Here's the drawing with two shaded views (mm, measured from the low corner). I have some questions. Coordinates: 2 decimals unless noted, no trailing zeros. Write each loop counter-clockwise with the first axis right and the second up, starting at its lowest first coordinate (ties: lowest second). Pieces come first, ordered by that corner, then holes.
Item 1: If we section it at A-A (x = 87.75): Please give me the cut outline in (y, z), then the cut area to 3 significant figures.
Item 2: If I drill on line 1 (Y direction, x = 87.75, z = 1.05); line 2 (Y direction, x = 2.2, z = 0.7); line 3 (Y direction, x = 4.75, z = 0.4), over which ranges is the centre line in solid material (lowest first)?
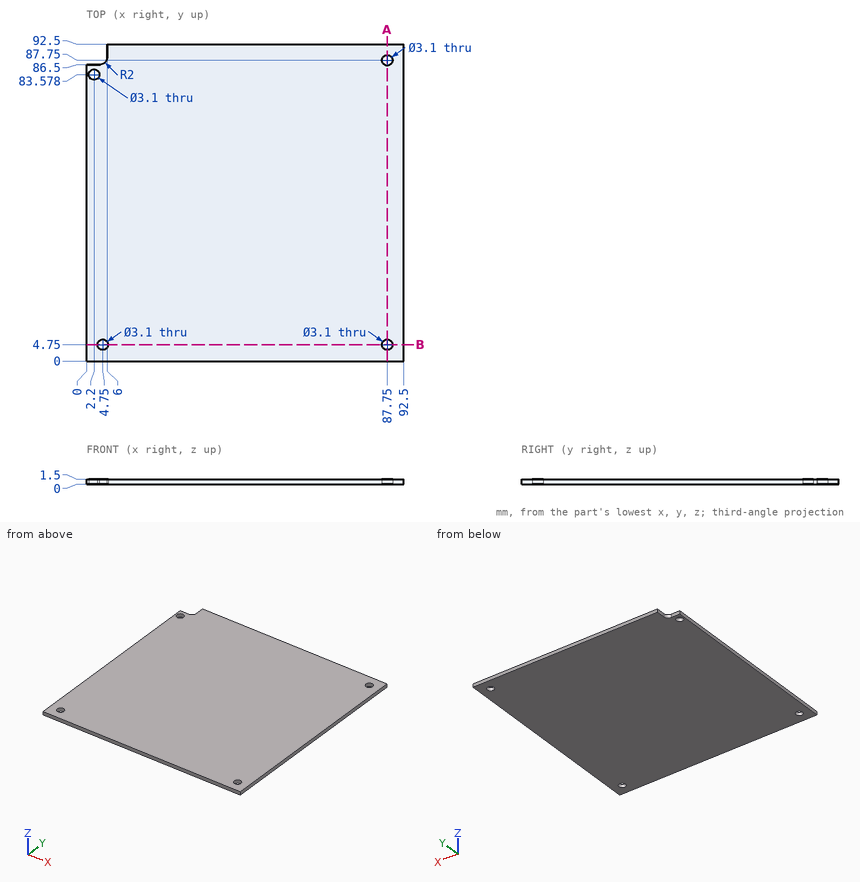
Answer list:
1. outline: (0, 0) - (3.2, 0) - (3.2, 1.5) - (0, 1.5) - close; (6.3, 0) - (86.2, 0) - (86.2, 1.5) - (6.3, 1.5) - close; (89.3, 0) - (92.5, 0) - (92.5, 1.5) - (89.3, 1.5) - close
1. area: 129 mm2
2. line 1: y = 0 to 3.2, 6.3 to 86.2, 89.3 to 92.5
2. line 2: y = 0 to 82.03, 85.13 to 86.5
2. line 3: y = 0 to 3.2, 6.3 to 86.65
